Here's the drawing with two shaded views (mm, measured from the low corner). I have some questions. A direction names the side the tool comes from. Round coordinates to 2 decimals unless told otherwise and drop trailing zeros. Loops run counter-clockwise (first coordinate to the right, second up) from the corner with the lowest first, then second, coordinate; pieces in that order, holes last.
(1) Thinking about a two-plate mould opening in Z: for the marked faces 1, 2, 3 and 4, which applies, released by +Z, released by -Z, zero draft, split by the parting line, or undercut?
(2) Which directions (+Z, -Z, +X, -X, +Y, -Y) give clear straight access to the entire face, cutting with the end or side of a thin tool? Please do the marked faces 5, 6 and 7.
(3) I want a section at A-A on y = 2. Write out the boundary of the cut face in (x, z), plus the area to 3 significant figures.
(4) I want a section at D-D on y = 9.25. Write out the boundary of the cut face in (x, z), plus the area to 3 significant figures.
(5) Will these pins go through, and if not, where does the flat tip stop? pin 1 Ø10 at (x, z) = (20, 9.5) entering from -Y; pin 2 Ø6.5 at (y, z) = (3.5, 11.5) entering from +X; pin 3 Ø4 at (x, z) = (8.5, 10.5) entering from -Y.
(6) I want a section at C-C on z = 17.5. Write out the boundary of the cut face in (x, y).
(7) If I drill on line 1 along Z through (x, y) = (5.75, 3.5); line 2 along Y through (x, z) = (22.5, 19.5); line 3 along X through (y, z) = (11, 10.5), over which ranges is the centre line in solid material (lowest first)?
(8) I want a section at B-B on x = 7. Write out the boundary of the cut face in (y, z), plus the area to 3 significant figures.
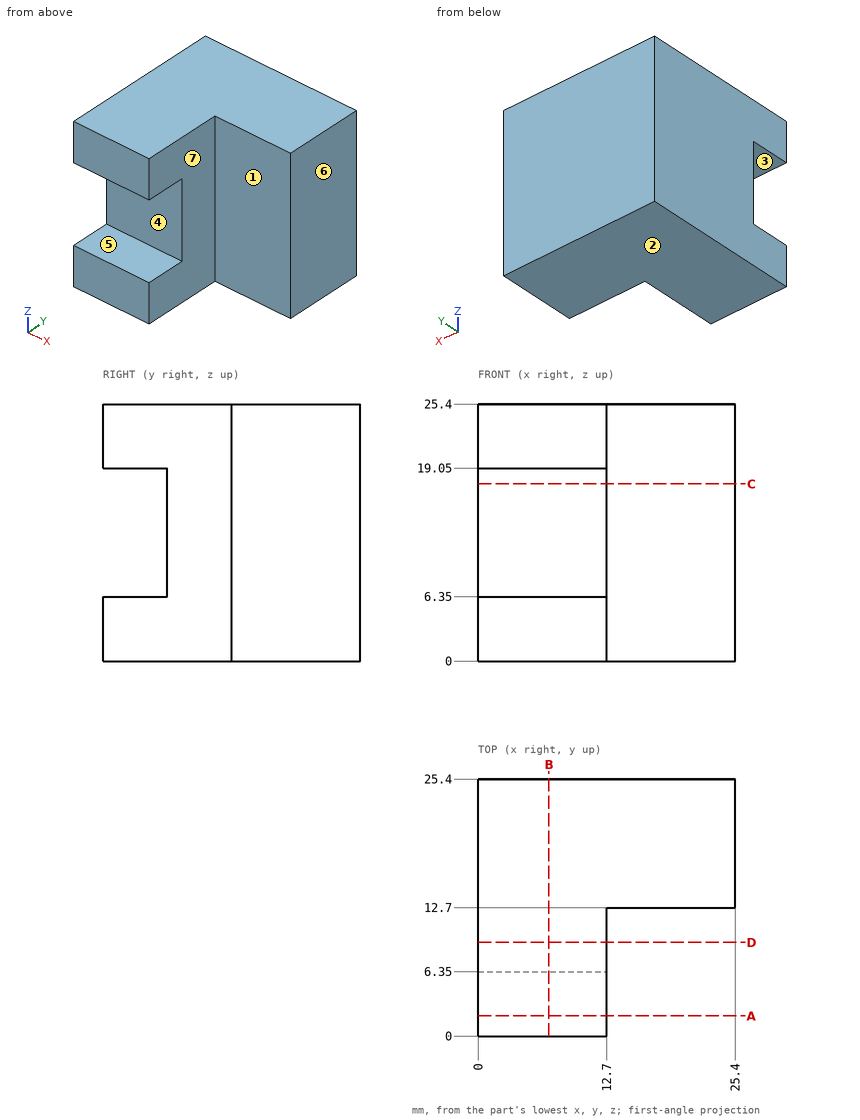
Filled sheet:
1. face 1: zero draft
1. face 2: released by -Z
1. face 3: undercut
1. face 4: undercut
2. face 5: +X, -X, -Y
2. face 6: +Z, -Z, +X, +Y, -Y
2. face 7: +Z, -Z, +X, -Y
3. outline: (0, 0) - (12.7, 0) - (12.7, 6.35) - (0, 6.35) - close; (0, 19.05) - (12.7, 19.05) - (12.7, 25.4) - (0, 25.4) - close
3. area: 161 mm2
4. outline: (0, 0) - (12.7, 0) - (12.7, 25.4) - (0, 25.4) - close
4. area: 323 mm2
5. pin 1: stops at y = 12.7
5. pin 2: stops at x = 12.7
5. pin 3: stops at y = 6.35
6. outline: (0, 6.35) - (12.7, 6.35) - (12.7, 12.7) - (25.4, 12.7) - (25.4, 25.4) - (0, 25.4) - close
7. line 1: z = 0 to 6.35, 19.05 to 25.4
7. line 2: y = 12.7 to 25.4
7. line 3: x = 0 to 12.7
8. outline: (0, 0) - (25.4, 0) - (25.4, 25.4) - (0, 25.4) - (0, 19.05) - (6.35, 19.05) - (6.35, 6.35) - (0, 6.35) - close
8. area: 565 mm2
